```python
from build123d import *

# Parameters (mm, degrees)
CUT_EXTRUDE1_START = 2
SKETCH2_W          = 4
SKETCH2_H          = 4
CUT_EXTRUDE1_DEPTH = 0.3


with BuildPart() as part:
    # Sketch1 → Revolve1 (revolve)
    with BuildSketch(Plane.XY, mode=Mode.PRIVATE) as revolve1_sk:
        Polygon((21.5, 0), (-21.5, 0), (-21.5, 2), (-20, 2), (-20, 1.5), (-19.5, 1.5), (-19.5, 2), (21.5, 2), align=None)
    revolve(revolve1_sk.sketch.rotate(Axis((-21.5, 0, 0), (-1, 0, 0)), 90), axis=Axis((-21.5, 0, 0), (-1, 0, 0)))

    # Sketch2 → Cut-Extrude1 (cut)
    with BuildSketch(Plane(origin=(0, 0, 0), x_dir=(1, 0, 0), z_dir=(0, 1, 0)).offset(CUT_EXTRUDE1_START)):
        with Locations((18, 0)):
            Rectangle(SKETCH2_W, SKETCH2_H)
    extrude(amount=-CUT_EXTRUDE1_DEPTH, mode=Mode.SUBTRACT)


solid = part.part
```
For this review, take the finished solid that the model builds, in its own axes (mm). Coordinates: 2 decimals unless noted, no trailing zeros. Loops run counter-clockwise (first coordinate to the right, second up) from the corner with the lowest first, then second, coordinate; pieces in that order, holes last. Notation, with made-up numbers: (52.25, 32) -> (101.25, 32) arc R14 ccw to (101.25, 37) -> close; hole circle Ø4 at (37, 1). An arc over 180 degrees is marked (long way). Return JSON: item names as keys, results as strings. Group by question number.
(1) Mouldability with a two-part tool opening along X and no side actions: class faces 1 (the cylindrical face through (1, -2, 0)), 2 (the flat face through (-21.5, 0, 0)), 3 (the flat face through (18, 1.7, 0)), 4 (the cylindrical face through (-19.75, -0.45, -1.43)) as pulls with the +X half, pulls with the -X half, needs draft (parallel to the pull), parting line crosses it, or undercut.
(2) Consider section C-C, the plane x = 19.5. Give the boundary of the cut face in (y, z).
(3) Consider section A-A, the plane y = -0.85. Give the boundary of the cut face in (x, z).
(4) To check wall thickness, follow L1, parallel to X at y = -1.8, z = -0.4; L2, parallel to Y at x = -11, z = 1.7; L3, parallel to Z at x = -2, y = -0.15. State the ranges of each line that lie inside material, in increasing order.
(5) For pin 1 Ø1.5 at (x, z) = (13, 1.5) entering from -Y; pin 2 Ø1.7 at (x, z) = (18, 0) entering from +Y; pin 3 Ø1.5 at (x, z) = (-5.5, -1.5) entering from +Y, all flat-tipped, find the tip position at first contact; note any pin that passes through.
(6) Consider section B-B, the plane x = -11. Give the boundary of the cut face in (y, z), plus the area to 3 significant figures.
Results below:
{
 "1": {"face 1": "needs draft", "face 2": "pulls with the -X half", "face 3": "undercut", "face 4": "undercut"},
 "2": {"outline": "(1.7, -1.05) -> (1.7, 1.05) arc R2 ccw (long way) to start"},
 "3": {"outline": "(-21.5, -1.81) -> (-20, -1.81) -> (-20, -1.24) -> (-19.5, -1.24) -> (-19.5, -1.81) -> (21.5, -1.81) -> (21.5, 1.81) -> (-19.5, 1.81) -> (-19.5, 1.24) -> (-20, 1.24) -> (-20, 1.81) -> (-21.5, 1.81) -> close"},
 "4": {"L1": "x = -21.5 to -20, -19.5 to 21.5", "L2": "y = -1.05 to 1.05", "L3": "z = -1.99 to 1.99"},
 "5": {"pin 1": "stops at y = -1.85", "pin 2": "stops at y = 1.7", "pin 3": "stops at y = 1.85"},
 "6": {"outline": "circle Ø4 at (0, 0)", "area": "12.6 mm2"}
}
